Drawing for the job (mm, zero at the part's lowest x, y, z). A direction names the side the tool comes from. Give positions to 0.01 mm unless a question says otherwise; leave off trailing zeros. Order: outer loops, then holes, each group sorted by start corner. A loop starts at its lowest first (then second) coordinate and runs counter-clockwise, first axis right, second up. Notation, with made-up numbers: (66.25, 17.5) -> (120.25, 17.5) arc R28 cw to (120.25, 56.5) -> close; hole circle Ø6 at (72.5, -28.5). An arc over 180 degrees is marked (long way). One line per item, written item: value. Start each with the question number.
(1) Saw through at A-A on x = 38.5. Give the cut face in (y, z), plus the area to 3 significant figures.
(2) Saw through at D-D on x = 57.5. Give the cut face in (y, z), plus the area to 3 significant figures.
(3) Which spindle directions (+Z, -Z, +X, -X, +Y, -Y) get a long thin tool onto all of the face, cutting with end or side? Do the marked faces 1, 2, 3 and 4. Say none if no direction does.
(4) Pin check, flat tips, straight feed: pin 1 (1 mm diameter, centred on x = 23, z = 12.5, fed in from -Y); pin 2 (12.5 mm diameter, centred on x = 19, y = 36.5, fed in from +Z); pin 3 (7.5 mm diameter, centred on y = 37.5, z = 39.5, fed in from +X); pin 4 (3 mm diameter, centred on y = 39, z = 15, fed in from -X). Stop position of each tip, or through.
(5) Two-plate mould, pull along X, no slides. Class the marked faces 5, 6, 7 and 8: +X half, -X half, draft (parallel to the pull), parting line (faces both ways), or undercut.
(6) Probe line 1 (Z direction, x = 64, y = 28); line 2 (X direction, y = 41.5, z = 56); line 3 (Z direction, x = 24.5, y = 17). List the from-to ranges inside material, lowest first.
(7) Saw through at B-B on y = 26.5. Give the cut face in (x, z), plus the area to 3 significant figures.
(8) Saw through at C-C on z = 37. Give the cut face in (x, y).
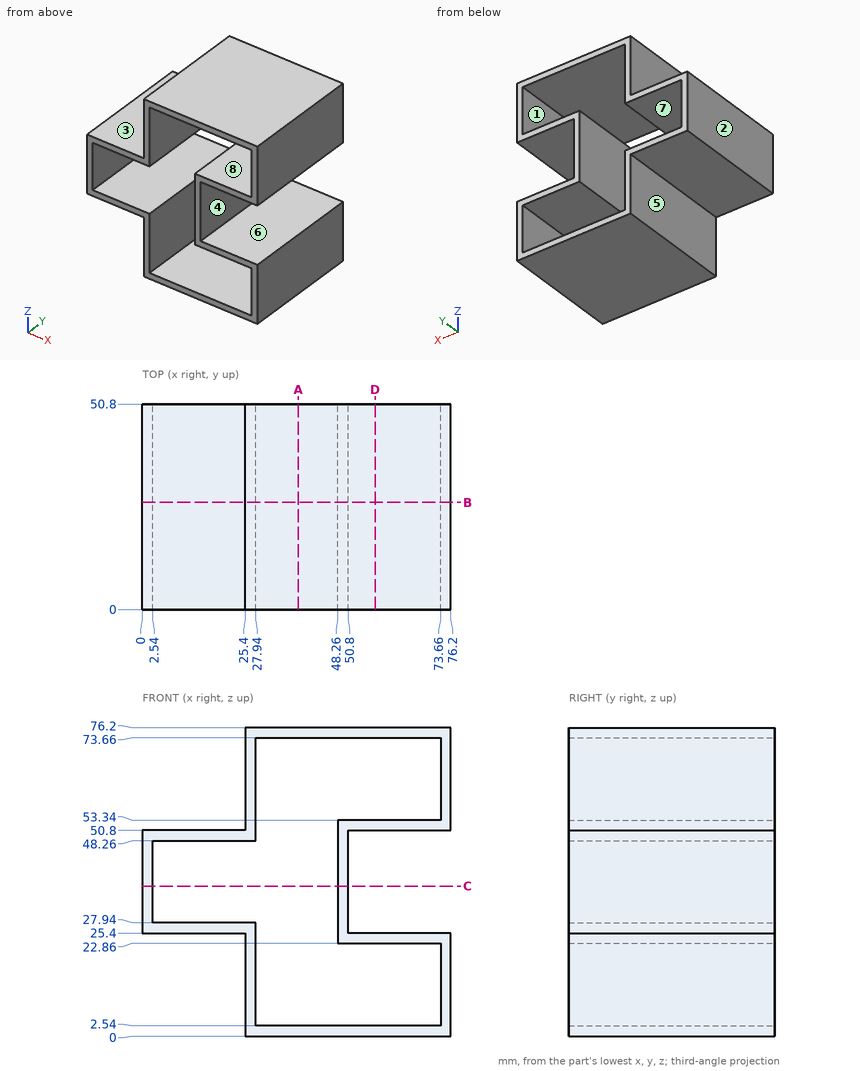
Results below:
1. outline: (0, 0) -> (50.8, 0) -> (50.8, 2.54) -> (0, 2.54) -> close; (0, 73.66) -> (50.8, 73.66) -> (50.8, 76.2) -> (0, 76.2) -> close
1. area: 258 mm²
2. outline: (0, 0) -> (50.8, 0) -> (50.8, 2.54) -> (0, 2.54) -> close; (0, 22.86) -> (50.8, 22.86) -> (50.8, 25.4) -> (0, 25.4) -> close; (0, 50.8) -> (50.8, 50.8) -> (50.8, 53.34) -> (0, 53.34) -> close; (0, 73.66) -> (50.8, 73.66) -> (50.8, 76.2) -> (0, 76.2) -> close
2. area: 516 mm²
3. face 1: +Y, -Y
3. face 2: +Z, -Z, -X, +Y, -Y
3. face 3: +Z, -X, +Y, -Y
3. face 4: +X, +Y, -Y
4. pin 1: passes through
4. pin 2: stops at z = 50.8
4. pin 3: stops at x = 50.8
4. pin 4: stops at x = 25.4
5. face 5: -X half
5. face 6: draft
5. face 7: undercut
5. face 8: undercut
6. line 1: z = 0 to 2.54, 22.86 to 25.4, 50.8 to 53.34, 73.66 to 76.2
6. line 2: x = 25.4 to 27.94, 73.66 to 76.2
6. line 3: z = 25.4 to 27.94, 48.26 to 50.8
7. outline: (0, 25.4) -> (25.4, 25.4) -> (25.4, 0) -> (76.2, 0) -> (76.2, 25.4) -> (50.8, 25.4) -> (50.8, 50.8) -> (76.2, 50.8) -> (76.2, 76.2) -> (25.4, 76.2) -> (25.4, 50.8) -> (0, 50.8) -> close; hole (2.54, 27.94) -> (27.94, 27.94) -> (27.94, 2.54) -> (73.66, 2.54) -> (73.66, 22.86) -> (48.26, 22.86) -> (48.26, 53.34) -> (73.66, 53.34) -> (73.66, 73.66) -> (27.94, 73.66) -> (27.94, 48.26) -> (2.54, 48.26) -> close
7. area: 877 mm²
8. outline: (0, 0) -> (2.54, 0) -> (2.54, 50.8) -> (0, 50.8) -> close; (48.26, 0) -> (50.8, 0) -> (50.8, 50.8) -> (48.26, 50.8) -> close
